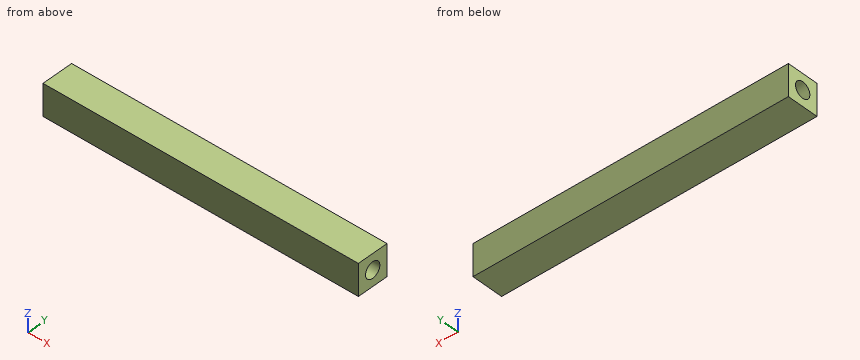
```python
from build123d import *

# Parameters (mm, degrees)
F0_W     = 76.2
F0_H     = 12.7
F1_DEPTH = 12.7
F2_R     = 3.175
F3_DEPTH = 85.27917
F4_DEPTH = 25.4
F5_DEPTH = 25.4


with BuildPart() as f1:
    # F0 (on Top) → F1 (new body)
    with BuildSketch(Plane.XY):
        with Locations((-38.1, -6.35)):
            Rectangle(F0_W, F0_H)
    extrude(amount=-F1_DEPTH)

    # F2 (on face) → F3 (cut)
    with BuildSketch(Plane.YZ):
        with Locations((-6.35, -6.35)):
            Circle(F2_R)
    extrude(amount=-F3_DEPTH, mode=Mode.SUBTRACT)

    # F4 (add): a face of the model
    f4_faces = [f1.faces().sort_by_distance(p)[0] for p in [
        (0, -12.5203948776, -6.35),
    ]]
    extrude(f4_faces, amount=F4_DEPTH)

    # F5 (add): a face of the model
    f5_faces = [f1.faces().sort_by_distance(p)[0] for p in [
        (-76.2, -0.1796051224, -6.35),
    ]]
    extrude(f5_faces, amount=F5_DEPTH)


solid = f1.part
```
Input: part model. Units: mm. Frame: model coordinates. Give positions to 0.01 mm unless a question says otherwise; leave off trailing zeros. Loops run counter-clockwise (first coordinate to the right, second up) from the corner with the lowest first, then second, coordinate; pieces in that order, holes last.
1) Contact query for a flat-ended pin moving along its axis: pin 1 (5.5 mm diameter, centred on y = -6.35, z = -6.35, fed in from +X). Output: stop coordinate, or through.
A:
pin 1: passes through
2) Section query C-C on x = -91. Return the cut outline in (y, z) (3 decimals), and give its area (3 significant figures).
A:
outline: (-12.7, -12.7) - (0, -12.7) - (0, 0) - (-12.7, 0) - close; hole circle Ø6.35 at (-6.35, -6.35)
area: 130 mm2
3) Section query A-A on z = -6.35. Return the cut outline in (x, y) (3 decimals).
A:
outline: (-101.6, -12.7) - (25.4, -12.7) - (25.4, -9.525) - (-101.6, -9.525) - close; (-101.6, -3.175) - (25.4, -3.175) - (25.4, 0) - (-101.6, 0) - close
4) Line query: L1, parallel to Z at x = -36, y = -6.35 (3 decimals); L2, parallel to Y at x = -57, z = -6.75; L3, parallel to Y at x = -5, z = -4.25. Output: solid intervals per line, ascending.
A:
L1: z = -12.7 to -9.525, -3.175 to 0
L2: y = -12.7 to -9.5, -3.2 to 0
L3: y = -12.7 to -8.73, -3.97 to 0
